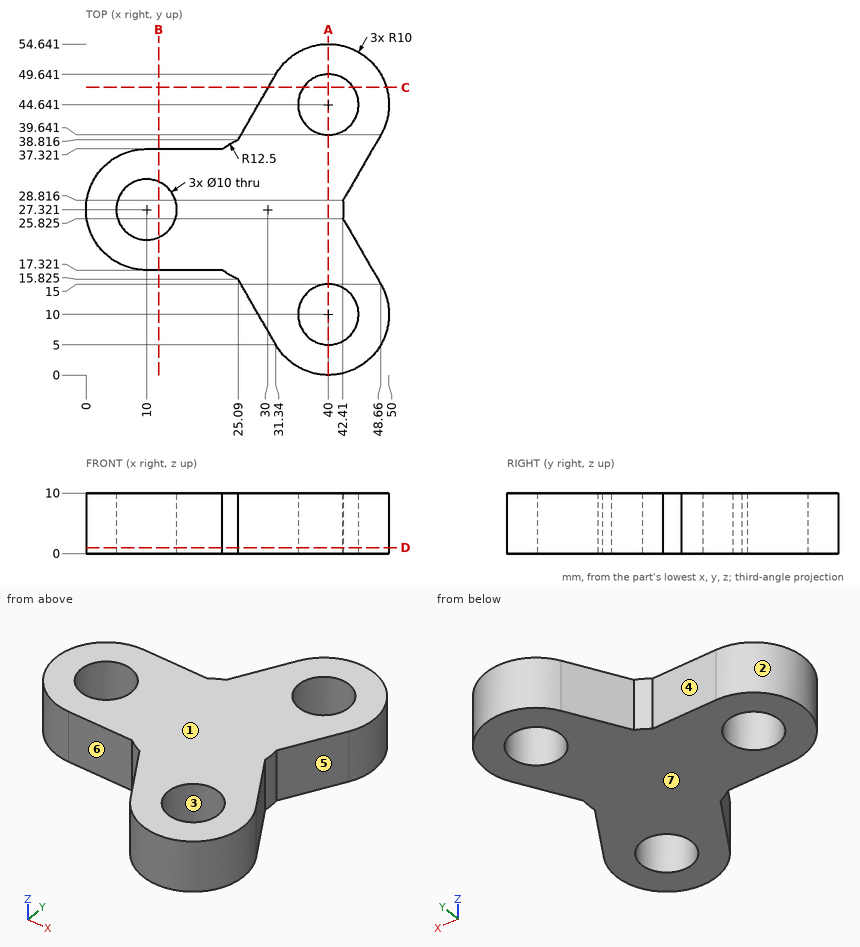
Job drawing, mm, ordinate dimensions from the low corner. One solid piece. A direction names the side the tool comes from. Give positions to 0.01 mm unless a question says otherwise; leave off trailing zeros. Loops run counter-clockwise (first coordinate to the right, second up) from the corner with the lowest first, then second, coordinate; pieces in that order, holes last. Notation, with made-up numbers: (-27.5, -12.5) -> (6.5, -12.5) arc R14 cw to (6.5, 9.5) -> close; hole circle Ø11 at (-7, -34). An arc over 180 degrees is marked (long way). Use a Markdown table: item, result. Add a question column.
(1) Wall check: line 1 along Y through (x, z) = (40, 7); line 2 along Y through (x, z) = (41.5, 2.75); line 3 along Y through (x, z) = (10, 7.5). Give the ranges that are in metal, low to high.
(2) Mould opens along Y. For the marked faces 1, 2 and 3 say: +Y half, -Y half, draft (parallel to the pull), parting line (faces both ways), or undercut.
(3) Slice it at B-B on x = 12. List the corners of the cut face in (y, z), and give its area (3 significant figures).
(4) Drop flat-ended pins along their axis: pin 1 Ø3 at (x, y) = (23.5, 12) entering from +Z (1 decimal); pin 2 Ø1 at (x, z) = (37, 3) entering from -Y; pin 3 Ø3 at (x, z) = (17.5, 6.5) entering from -Y. Give the stop position or say it passes through.
(5) Slice it at D-D on z = 1. List the corners of the cut face in (x, y) (1 decimal), and give its area (3 significant figures).
(6) Tool access for the marked faces 4, 5, 6 and 7: list every direction of +Z, -Z, +X, -X, +Y, -Y with a clear straight run to the whole face (end or side of a thin tool).
(7) Slice it at A-A on x = 40. List the corners of the cut face in (y, z).
(8) Slice it at C-C on y = 47.5. List the corners of the cut face in (x, z).
Filled sheet:
| question | item | result |
|---|---|---|
| 1 | line 1 | 0 to 5, 15 to 39.64, 49.64 to 54.64 |
| 1 | line 2 | 0.11 to 5.23, 14.77 to 39.87, 49.41 to 54.53 |
| 1 | line 3 | 17.32 to 22.32, 32.32 to 37.32 |
| 2 | face 1 | draft |
| 2 | face 2 | parting line |
| 2 | face 3 | undercut |
| 3 | outline | (17.32, 0) -> (22.74, 0) -> (22.74, 10) -> (17.32, 10) -> close; (31.9, 0) -> (37.32, 0) -> (37.32, 10) -> (31.9, 10) -> close |
| 3 | area | 108 mm2 |
| 4 | pin 1 | through |
| 4 | pin 2 | y = 0.32 |
| 4 | pin 3 | y = 17.32 |
| 5 | outline | (10, 17.3) -> (22.5, 17.3) arc R12.5 ccw to (25.1, 15.8) -> (31.3, 5) arc R10 ccw to (48.7, 15) -> (42.4, 25.8) arc R12.5 ccw to (42.4, 28.8) -> (48.7, 39.6) arc R10 ccw to (31.3, 49.6) -> (25.1, 38.8) arc R12.5 ccw to (22.5, 37.3) -> (10, 37.3) arc R10 ccw to start; hole circle Ø10 at (10, 27.3); hole circle Ø10 at (40, 10); hole circle Ø10 at (40, 44.6) |
| 5 | area | 1,270 mm2 |
| 6 | face 4 | +Z, -Z, -X, +Y |
| 6 | face 5 | +Z, -Z, +X |
| 6 | face 6 | +Z, -Z, -X, -Y |
| 6 | face 7 | -Z, +X, -X, +Y, -Y |
| 7 | outline | (0, 0) -> (5, 0) -> (5, 10) -> (0, 10) -> close; (15, 0) -> (39.64, 0) -> (39.64, 10) -> (15, 10) -> close; (49.64, 0) -> (54.64, 0) -> (54.64, 10) -> (49.64, 10) -> close |
| 8 | outline | (30.1, 0) -> (35.9, 0) -> (35.9, 10) -> (30.1, 10) -> close; (44.1, 0) -> (49.58, 0) -> (49.58, 10) -> (44.1, 10) -> close |
